Work out the finished part from the listing and answer in its coordinate system (mm). Round coordinates to 2 decimals unless told otherwise and drop trailing zeros. Write each loop counter-clockwise with the first axis right and the second up, starting at its lowest first coordinate (ties: lowest second). Pieces come first, ordered by that corner, then holes. Notation, with made-up numbers: (-36.75, -34.5) -> (-7.75, -34.5) arc R16 ccw to (-7.75, -26.5) -> close; hole circle Ø9 at (-37.75, 57). An arc over 180 degrees is marked (long way). One line per item, written item: value.
```python
from build123d import *

# Parameters (mm, degrees)
BOSS_EXTRUDE1_DEPTH  = 5
CUT_EXTRUDE1_DEPTH   = 10
MIRROR2_COPY_1_DEPTH = 10
SKETCH4_W            = 5
SKETCH4_H            = 15
CUT_EXTRUDE2_DEPTH   = 10


with BuildPart() as part:
    # Sketch2 → Boss-Extrude1 (new body)
    with BuildSketch(Plane.XY):
        Polygon((-10, 100), (-35, 100), (-35, -100), (-10, -100), (-10, -95), (10, -95), (10, -100), (35, -100), (35, 100), (10, 100), (10, 95), (-10, 95), align=None)
    extrude(amount=BOSS_EXTRUDE1_DEPTH)

    # Sketch3 → Cut-Extrude1 (cut)
    with BuildSketch(Plane.XY.offset(5)):
        Polygon((35, -52), (29, -52), (29, -53.5), (25, -53.5), (25, -52), (23, -52), (23, -48), (25, -48), (25, -46.5), (29, -46.5), (29, -48), (35, -48), align=None)
    cut_extrude1 = extrude(amount=-CUT_EXTRUDE1_DEPTH, mode=Mode.SUBTRACT)

    # Mirror1: Cut-Extrude1 across plane
    add(cut_extrude1.mirror(Plane.ZX), mode=Mode.SUBTRACT)

    # Mirror2: Cut-Extrude1 across plane
    add(cut_extrude1.mirror(Plane(origin=(0, 0, 0), x_dir=(0, 0, 1), z_dir=(1, 0, 0))), mode=Mode.SUBTRACT)

    # Mirror2 copy 1 sketch → Mirror2 copy 1 (cut)
    with BuildSketch(Plane(origin=(0, 0, 5), x_dir=(-1, 0, 0), z_dir=(0, 0, 1))):
        Polygon((35, -52), (29, -52), (29, -53.5), (25, -53.5), (25, -52), (23, -52), (23, -48), (25, -48), (25, -46.5), (29, -46.5), (29, -48), (35, -48), align=None)
    extrude(amount=-MIRROR2_COPY_1_DEPTH, mode=Mode.SUBTRACT)

    # Sketch4 → Cut-Extrude2 (cut)
    with BuildSketch(Plane(origin=(0, 0, 0), x_dir=(-1, 0, 0), z_dir=(0, 0, -1))):
        with Locations((-32.5, -60)):
            Rectangle(SKETCH4_W, SKETCH4_H)
    extrude(amount=-CUT_EXTRUDE2_DEPTH, mode=Mode.SUBTRACT)


solid = part.part
```
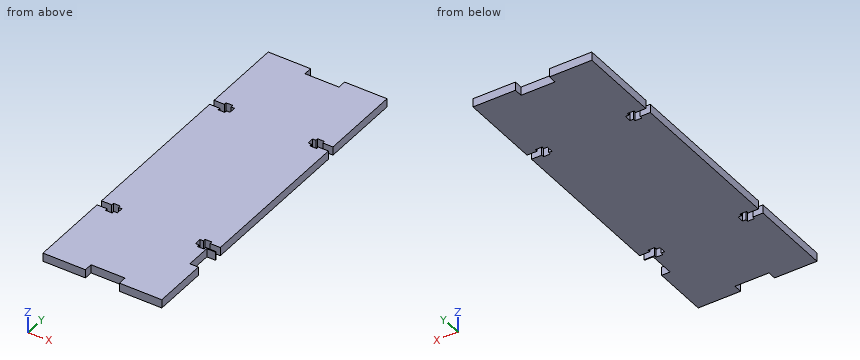
(1) Find section A-A on x = -1.5. Give the vertices of the cut face in (y, z), plus the area to 3 significant figures.
Reported:
outline: (-95, 0) -> (95, 0) -> (95, 5) -> (-95, 5) -> close
area: 950 mm2
(2) Consider probe 1 along Y at (x, z) = (-26.5, 1.2); probe 2 along X at (y, z) = (47, 4.2); probe 3 along Y at (x, z) = (23.5, 1.9). Determine where each line is inside the solid, lowest interval first.
Reported:
probe 1: y = -100 to -53.5, -46.5 to 46.5, 53.5 to 100
probe 2: x = -35 to -29, -25 to 25, 29 to 35
probe 3: y = -100 to -52, -48 to 48, 52 to 100
(3) Find section B-B on y = -55.5. Give the vertices of the cut face in (x, z), plus the area to 3 significant figures.
Reported:
outline: (-35, 0) -> (30, 0) -> (30, 5) -> (-35, 5) -> close
area: 325 mm2
(4) A flat-ended cylindrical pin translates along its axis: pin 1 Ø1 at (x, z) = (-2, 2.5) entering from +Y. Find the tip coordinate at first contact, or state that the pin passes through.
Reported:
pin 1: stops at y = 95
